Autodesk Inventor part; units mm, degrees
ref_plane "工作平面5" through (-8, 0, 4.5) normal (0, 0, 1) x (1, 0, 0)
ref_plane "工作平面2" through (-8, 0, 7.5) normal (0, 0, 1) x (1, 0, 0)
ref_plane "YZ Plane" through (0, 0, 0) normal (1, 0, 0) x (0, 1, 0)
ref_plane "工作平面5" through (-8, 0, 4.5) normal (0, 0, 1) x (1, 0, 0)
sketch "草图5" plane through (-8, 0, 4.5) normal (0, 0, 1) x (1, 0, 0)
  arc A0 (-229.373, 177.0271) -> (-229.1311, 177.052) centre (-230.6821, 190.9658) ccw
  circle A1 centre (-229.4321, 193.1309) radius 6
  circle A2 centre (-177.5679, 193.1309) radius 6
  circle A3 centre (-203.5, 148.2151) radius 6
  arc A4 (-172.5679, 184.4706) -> (-182.5679, 201.7911) centre (-177.5679, 193.1309) ccw
  arc A5 (-224.4321, 201.7911) -> (-234.4321, 184.4706) centre (-229.4321, 193.1309) ccw
  arc A6 (-213.5, 148.2151) -> (-193.5, 148.2151) centre (-203.5, 148.2151) ccw
  line L0 (-234.4321, 184.4706) -> (-218.5, 175.2722)
  line L1 (-172.5679, 184.4706) -> (-188.5, 175.2722)
  line L2 (-224.4321, 201.7911) -> (-208.5, 192.5927)
  line L3 (-182.5679, 201.7911) -> (-198.5, 192.5927)
  line L4 (-213.5, 148.2151) -> (-213.5, 166.6119)
  line L5 (-193.5, 148.2151) -> (-193.5, 166.6119)
  line L6 (-206, 177.7999) -> (-206, 178.2297)
  arc A7 (-208.5, 192.5927) -> (-198.5, 192.5927) centre (-203.5, 201.2529) ccw
  arc A8 (-188.5, 175.2722) -> (-193.5, 166.6119) centre (-183.5, 166.6119) ccw
  arc A9 (-213.5, 166.6119) -> (-218.5, 175.2722) centre (-223.5, 166.6119) ccw
  point P0 (8, 0)
  point P1 (-184.4262, 177.6242)
  point P2 (-222.5767, 177.6259)
  dimension "d31" = 12
  dimension "d33" = 12
  dimension "d37" = 20
  dimension "d38" = 20
  dimension "d44" = 10
  dimension "d87" = 12
extrude "拉伸1" add sketch "草图5" along normal blind 3
ref_plane "工作平面2" through (-8, 0, 7.5) normal (0, 0, 1) x (1, 0, 0)
sketch "草图8" plane through (-8, 0, 4.5) normal (0, 0, -1) x (-1, 0, 0)
  circle A0 centre (203.5, 148.2151) radius 6
  circle A1 centre (203.5, 148.2151) radius 6
  circle A2 centre (229.4321, 193.1309) radius 6
  circle A3 centre (229.4321, 193.1309) radius 6
  circle A4 centre (177.5679, 193.1309) radius 6
  circle A5 centre (177.5679, 193.1309) radius 6
  point P0 (-8, 0)
sketch "草图9" plane through (-8, 0, 4.5) normal (0, 0, -1) x (-1, 0, 0)
  point P0 (-8, 0)
extrude "拉伸3" add sketch "草图8" against normal blind 37
hole "孔4" at (-237.4321, 193.1309, 41.5) direction (0, 0, -1) diameter 1.941 depth 10 tip angle 118
hole "孔5" at (-185.5679, 193.1309, 41.5) direction (0, 0, -1) diameter 1.941 depth 10 tip angle 118
hole "孔6" at (-211.5, 148.2151, 41.5) direction (0, 0, -1) diameter 1.941 depth 10 tip angle 118
fillet "圆角4" radius 0.3 3 edges at (-231.4321, 193.1309, 41.5) (-179.5679, 193.1309, 41.5) (-205.5, 148.2151, 41.5)
sketch "草图10" plane through (-8, 0, 4.5) normal (0, 0, -1) x (-1, 0, 0)
  circle A0 centre (229.4321, 193.1309) radius 6
  circle A1 centre (203.5, 148.2151) radius 6
  circle A2 centre (177.5679, 193.1309) radius 6.4097
  point P0 (-8, 0)
extrude "拉伸4" cut sketch "草图10" against normal blind 1
equation "\"折弯半径\" = 厚度"
equation "\"折弯释压宽度\" = 厚度"
equation "\"折弯释压深度\" = 0.5 * 厚度"
equation "\"拐角释压尺寸\" = 4 * 厚度"
equation "\"最小余量\" = 2 * 厚度"
equation "\"过渡半径\" = 折弯半径"
equation "\"Jacobi半径尺寸\" = 折弯半径"
equation "\"间隙大小\" = 厚度"
Source: CAD feature listing. Evaluate the final solid. Frame: model axes, mm. A direction names the side the tool comes from. Coordinates: 2 decimals unless noted, no trailing zeros. Loops run counter-clockwise (first coordinate to the right, second up) from the corner with the lowest first, then second, coordinate; pieces in that order, holes last. Notation, with made-up numbers: (85, 11.25) -> (104, 11.25) arc R17 ccw to (104, 31.25) -> close; hole circle Ø7 at (-17, 49.25). An arc over 180 degrees is marked (long way). One line per item, written item: value. Start each with the question number.
Q1. Section query B-B, the plane z = 28. Return the cut outline in (x, y), and give its area (3 significant figures).
Q2. Section query C-C, the plane y = 156. Return the cut outline in (x, z), and give its area (3 significant figures).
Q3. Section query D-D, the plane x = -220.5. Return the cut outline in (y, z).
Q4. Set-up query: faces 4 (the face through (-200.197, 171.548, 5.979)), 5 (the face through (-211.79, 147.29, 36.43)), 6 (the face through (-191.5, 190.7, 5)), 7 (the face through (-221.5, 157, 6)), 8 (the face through (-198.422, 197.256, 5.979)). Return all of +Z, -Z, +X, -X, +Y, -Y with unobstructed straight access to the full face (end or side cutting, diameter ignored); none if empty.
Q5. Mould query, pull axis Y, two halves, no side actions, for faces 1 (the face through (-211.427, 191.253, 5.979)), 2 (the face through (-185.52, 192.97, 31.02)), 3 (the face through (-211, 147, 41.5)). Classes: pulls with the +Y half, pulls with the -Y half, needs draft (parallel to the pull), parting line crosses it, or undercut.
Q6. Contact query for flat-ended pins moving along their axis: P1, Ø3, axis at x = -187.5, z = 28, coming from the +Y side; P2, Ø1, axis at y = 176.5, z = 9.5, coming from the -X side; P3, Ø11.5, axis at x = -185.57, y = 193.13, coming from the -Z side; P4, Ø1.6, axis at x = -185.57, y = 193.13, coming from the +Z side. Output: stop coordinate, or through.
Q7. Section query A-A, the plane z = 35.5. Return the cut outline in (x, y).
Q8. Line query: line 1 along Z through (x, y) = (-204, 164.5); line 2 along Z through (x, y) = (-187, 191); line 3 along X through (y, z) = (198, 35). Output: solid intervals per line, ascending.
Results:
1. outline: circle Ø12 at (-237.43, 193.13); circle Ø12 at (-211.5, 148.22); circle Ø12 at (-185.57, 193.13)
1. area: 339 mm^2
2. outline: (-221.5, 4.5) -> (-201.5, 4.5) -> (-201.5, 7.5) -> (-221.5, 7.5) -> close
2. area: 60.0 mm^2
3. outline: (143.86, 4.5) -> (194.9, 4.5) -> (194.9, 7.5) -> (143.86, 7.5) -> close
4. face 4: +Z, -Z, +X, -Y
4. face 5: +Z
4. face 6: -Z
4. face 7: +Z, -Z, -X, -Y
4. face 8: +Z, -Z, +Y
5. face 1: pulls with the +Y half
5. face 2: undercut
5. face 3: needs draft
6. P1: y = 199.12
6. P2: through
6. P3: z = 5.5
6. P4: z = 31.4
7. outline: circle Ø12 at (-237.43, 193.13); circle Ø12 at (-211.5, 148.22); circle Ø12 at (-185.57, 193.13); hole circle Ø1.94 at (-237.43, 193.13); hole circle Ø1.94 at (-211.5, 148.22); hole circle Ø1.94 at (-185.57, 193.13)
8. line 1: 4.5 to 7.5
8. line 2: 5.5 to 41.5
8. line 3: -240.94 to -233.93, -189.07 to -182.06
